Here's how the part is built. I have some questions about the finished solid (model axes, mm). A direction names the side the tool comes from. Coordinates: 2 decimals unless noted, no trailing zeros. Loops run counter-clockwise (first coordinate to the right, second up) from the corner with the lowest first, then second, coordinate; pieces in that order, holes last. Notation, with made-up numbers: M -23.75,55 L 30.25,55 A28 ccw 30.25,83 Z; hole C 74.5,-4 d8. An arc over 180 degrees is marked long. Use CSV: the item, a comma, the result in double quotes. Start each with the question number.
Q1. If we section it at B-B (z = 0): Please give me the cut outline in (x, y).
Q2. Which directions (+Z, -Z, +X, -X, +Y, -Y) give clear straight access to the entire face, cutting with the end or side of a thin tool? Please do faces 1 (the cylindrical face through (-7.974, 2.218, -13.053)), 2 (the flat face through (-7, 4.5, -13)).
Q3. If we section it at C-C (y = 7.5): Please give me the cut outline in (x, z).
Q4. If we section it at D-D (y = 0.75): Please give me the cut outline in (x, z).
Q5. For pin 1 Ø4 at (x, y) = (-2.5, 6) entering from +Z; pin 2 Ø1.5 at (x, y) = (14.5, 2.5) entering from +Z; pin 3 Ø6 at (x, z) = (-8.5, 14.72) entering from +Y, each with a flat end and sliding along its axis, tell me the tip position at first contact or that it passes through.
Q6. Please list where these lines run through material, in increasing order: probe 1 along Z at (x, y) = (-7, 5.25) (3 decimals); probe 2 along X at (y, z) = (2, -2); probe 3 along Z at (x, y) = (17, 2.4). Write a range as [from, to].
Q7. If we section it at A-A (x = 0): Please give me the cut outline in (y, z), and give its area (3 significant figures).
from build123d import *

# Parameters (mm, degrees)
SKETCH1_R           = 20
SKETCH1_R_2         = 1.75
BOSS_EXTRUDE1_DEPTH = 8
SKETCH2_R           = 3.25
CUT_EXTRUDE1_DEPTH  = 3.5
SKETCH3_R           = 2.54000508
CUT_EXTRUDE2_DEPTH  = 30.393876913
FILLET1_R           = 2


with BuildPart() as part:
    # Sketch1 → Boss-Extrude1 (new body)
    with BuildSketch(Plane(origin=(0, 0, 0), x_dir=(1, 0, 0), z_dir=(0, 1, 0))):
        with Locations(Location((0, 0, 0), (0, 0, 270))):
            Circle(SKETCH1_R)
        with Locations(Location((17, 0, 0), (0, 0, 270))):
            Circle(SKETCH1_R_2, mode=Mode.SUBTRACT)
        with Locations(Location((-8.5, -14.722431864, 0), (0, 0, 270))):
            Circle(SKETCH1_R_2, mode=Mode.SUBTRACT)
        with Locations(Location((-8.5, 14.722431864, 0), (0, 0, 270))):
            Circle(SKETCH1_R_2, mode=Mode.SUBTRACT)
    extrude(amount=BOSS_EXTRUDE1_DEPTH)

    # Sketch2 → Cut-Extrude1 (cut)
    with BuildSketch(Plane(origin=(0, 8, 0), x_dir=(1, 0, 0), z_dir=(0, 1, 0))):
        with Locations((17, 0)):
            Circle(SKETCH2_R)
        with Locations((-8.5, -14.722431864)):
            Circle(SKETCH2_R)
        with Locations((-8.5, 14.722431864)):
            Circle(SKETCH2_R)
    extrude(amount=-CUT_EXTRUDE1_DEPTH, mode=Mode.SUBTRACT)

    # Sketch3 → Cut-Extrude2 (cut, through all)
    with BuildSketch(Plane(origin=(0, 8, 0), x_dir=(1, 0, 0), z_dir=(0, 1, 0))):
        with Locations(Location((0, 0, 0), (0, 0, 270))):
            Circle(SKETCH3_R)
    extrude(amount=-CUT_EXTRUDE2_DEPTH, mode=Mode.SUBTRACT)

    # Fillet1
    fillet1_edges = [part.edges().sort_by_distance(p)[0] for p in [
        (10, 8, -17.320508076),
        (-20, 8, 0),
        (13.654656242, 8, 14.613362478),
    ]]
    fillet(fillet1_edges, radius=FILLET1_R)


solid = part.part
Results below:
1,outline,"M -20,0 L -2.54,0 L -2.54,8 L -18,8 A2 ccw -20,6 Z; M 2.54,0 L 15.25,0 L 15.25,4.5 L 13.75,4.5 L 13.75,8 L 2.54,8 Z; M 18.75,0 L 20,0 L 20,4.5 L 18.75,4.5 Z"
2,face 1,"+Y, -Y"
2,face 2,"+Y"
3,outline,"M -11.68,-15.39 A3.25 cw long -7.49,-17.81 A19.32 ccw 19.17,-2.42 A3.25 cw long 19.17,2.42 A19.32 ccw -7.49,17.81 A3.25 cw long -11.68,15.39 A19.32 ccw Z; hole C 0,0 d5.08"
4,outline,"C 0,0 d40; hole C -8.5,-14.72 d3.5; hole C -8.5,14.72 d3.5; hole C 0,0 d5.08; hole C 17,0 d3.5"
5,pin 1,"z = 19.99"
5,pin 2,"z = 14.52"
5,pin 3,"y = 4.5"
6,probe 1,"[-18.735, -17.606], [-11.839, 11.839], [17.606, 18.735]"
6,probe 2,"[-19.9, -1.57], [1.57, 19.9]"
6,probe 3,"[-10.54, -1.75], [1.75, 10.54]"
7,outline,"M 0,-20 L 6,-20 A2 ccw 8,-18 L 8,-2.54 L 0,-2.54 Z; M 0,2.54 L 8,2.54 L 8,18 A2 ccw 6,20 L 0,20 Z"
7,area,"278 mm^2"
